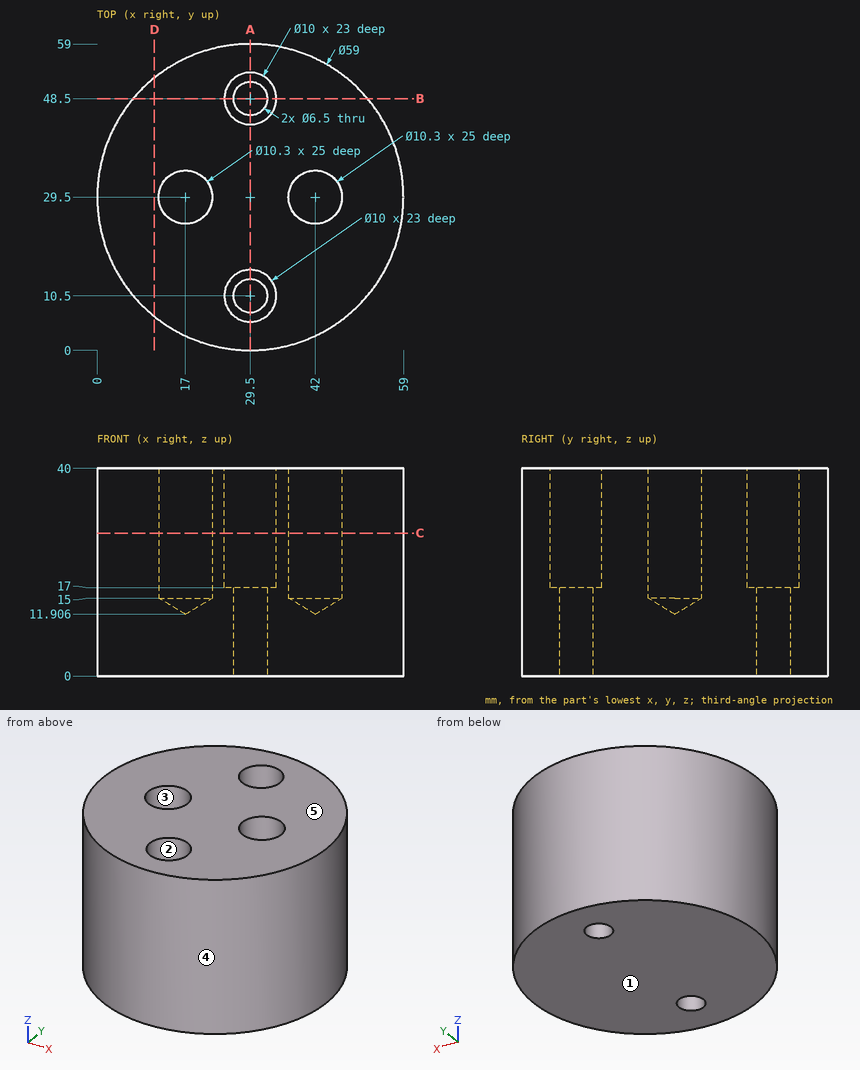
Could you check a few things on this drawing? It's one solid part, dimensions in mm from its lowest x, y, z. A direction names the side the tool comes from. Coordinates: 2 decimals unless noted, no trailing zeros. Order: outer loops, then holes, each group sorted by start corner. A loop starts at its lowest first (then second) coordinate and runs counter-clockwise, first axis right, second up.
1. I'm going to push flat-ended pins straight in: pin 1 (2 mm diameter, centred on x = 27, z = 19, fed in from -Y); pin 2 (4 mm diameter, centred on x = 12, z = 5.5, fed in from +Y); pin 3 (1 mm diameter, centred on x = 34, z = 32.5, fed in from -Y). Where does each tip first touch, or does it pass through?
2. Thinking about a two-plate mould opening in Y: for the marked faces 3, 4 and 5, which applies, +Y half, -Y half, draft (parallel to the pull), parting line (faces both ways), or undercut?
3. For the marked faces 1 and 2, which set-ups out of +Z, -Z, +X, -X, +Y, -Y let a thin tool reach every point of the face, with its end or its side?
4. If we section it at B-B (y = 48.5): Please give me the cut outline in (x, z), then the cut area to 4 significant figures.
5. If we section it at C-C (z = 27.5): Please give me the cut outline in (x, y).
6. If we section it at D-D (x = 11): Please give me the cut outline in (y, z).
7. I need wall thicknesses on line 1 (Y direction, x = 29.5, z = 5); line 2 (Y direction, x = 27, z = 18) (1 decimal); line 3 (Y direction, x = 19, z = 22) (1 decimal). Which ranges of each line are inside material? Lowest first, please.
8. If we section it at A-A (x = 29.5): Please give me the cut outline in (y, z), then the cut area to 3 significant figures.
Entries:
1. pin 1: stops at y = 0.04
1. pin 2: stops at y = 54.6
1. pin 3: stops at y = 0.27
2. face 3: undercut
2. face 4: parting line
2. face 5: draft
3. face 1: -Z, +X, -X, +Y, -Y
3. face 2: +Z
4. outline: (6.93, 0) - (26.25, 0) - (26.25, 17) - (24.5, 17) - (24.5, 40) - (6.93, 40) - close; (32.75, 0) - (52.07, 0) - (52.07, 40) - (34.5, 40) - (34.5, 17) - (32.75, 17) - close
4. area: 1,465 mm2
5. outline: circle Ø59 at (29.5, 29.5); hole circle Ø10.3 at (17, 29.5); hole circle Ø10 at (29.5, 10.5); hole circle Ø10 at (29.5, 48.5); hole circle Ø10.3 at (42, 29.5)
6. outline: (6.52, 0) - (52.48, 0) - (52.48, 40) - (6.52, 40) - close
7. line 1: y = 0 to 7.25, 13.75 to 45.25, 51.75 to 59
7. line 2: y = 0.1 to 6.2, 14.8 to 44.2, 52.8 to 58.9
7. line 3: y = 1.9 to 24.8, 34.2 to 57.1
8. outline: (0, 0) - (7.25, 0) - (7.25, 17) - (5.5, 17) - (5.5, 40) - (0, 40) - close; (13.75, 0) - (45.25, 0) - (45.25, 17) - (43.5, 17) - (43.5, 40) - (15.5, 40) - (15.5, 17) - (13.75, 17) - close; (51.75, 0) - (59, 0) - (59, 40) - (53.5, 40) - (53.5, 17) - (51.75, 17) - close
8. area: 1,680 mm2
